Could you check a few things on this model? Use its own coordinates, in mm. Face numbers are marked on the shaded views. A direction names the side the tool comes from. Give positions to 0.01 mm unless a question says otherwise; leave off trailing zeros. Write each loop counter-clockwise with the first axis right and the second up, starting at its lowest first coordinate (ties: lowest second). Pieces come first, ordered by that corner, then holes. Notation, with made-up numbers: M 29.5,-15 L 66.5,-15 A12 cw 66.5,6 Z; hole C -8.5,6.25 d5. An arc over 180 degrees is marked long. Use one line per item in the form item = value.
from build123d import *

# Parameters (mm, degrees)
F0_R      = 14.5
F1_DEPTH  = 2
F2_R      = 11
F3_DEPTH  = 20
F4_R      = 2.9
F5_DEPTH  = 22.001
F6_W      = 3
F6_H      = 3.4
F7_DEPTH  = 2
F8_R      = 0.8
F9_R      = 0.5
F11_W     = 28.85052
F11_H     = 54.144128
F12_DEPTH = 22.001
F14_W     = 3.5
F14_H     = 9


with BuildPart() as f1:
    # F0 (on Top) → F1 (new body)
    with BuildSketch(Plane.XY):
        Circle(F0_R)
    extrude(amount=F1_DEPTH)

    # F2 (on face) → F3 (join)
    with BuildSketch(Plane.XY.offset(2)):
        Circle(F2_R)
    extrude(amount=F3_DEPTH)

    # F4 (on face) → F5 (cut, through all)
    with BuildSketch(Plane(origin=(0, 0, 0), x_dir=(1, 0, 0), z_dir=(0, 0, -1))):
        Circle(F4_R)
    extrude(amount=-F5_DEPTH, mode=Mode.SUBTRACT)

    # F6 (on face) → F7 (join)
    with BuildSketch(Plane.XY.offset(2)):
        with Locations((0, -11)):
            Rectangle(F6_W, F6_H)
    extrude(amount=F7_DEPTH)

    # F8
    f8_edges = [f1.edges().sort_by_distance(p)[0] for p in [
        (-1.5, -12.7, 3),
        (1.5, -12.7, 3),
    ]]
    fillet(f8_edges, radius=F8_R)

    # F9
    f9_edges = [f1.edges().sort_by_distance(p)[0] for p in [
        (-11, 0, 22),
    ]]
    fillet(f9_edges, radius=F9_R)

    # F11 (on Top) → F12 (cut, through all)
    with BuildSketch(Plane.XY):
        with Locations((-14.42526, 2.568883)):
            Rectangle(F11_W, F11_H)
    extrude(amount=F12_DEPTH, mode=Mode.SUBTRACT)

    # F14 (on Front) → F15 (revolve, cut)
    with BuildSketch(Plane.XZ):
        with Locations((9.25, 13.5)):
            Rectangle(F14_W, F14_H)
    revolve(axis=Axis((0, 0, 13.307823), (0, 0, 1)), mode=Mode.SUBTRACT)


solid = f1.part
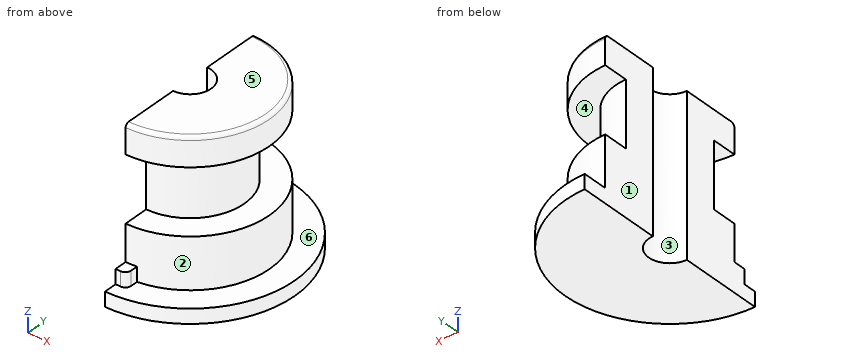
1) I want a section at A-A, the plane y = 0. Please give me the cut outline in (x, z), plus the area to 3 significant figures.
Checked values:
outline = M 2.9,0 L 14.5,0 L 14.5,2 L 11,2 L 11,9 L 7.5,9 L 7.5,18 L 11,18 L 11,21.5 A0.5 ccw 10.5,22 L 2.9,22 Z
area = 154 mm2
2) I want a section at C-C, the plane z = 14. Please give me the cut outline in (x, y).
Checked values:
outline = M 0,-7.5 A7.5 ccw 0,7.5 L 0,2.9 A2.9 cw 0,-2.9 Z
3) Thinking about a two-plate mould opening in Y: for the marked faces 1, 2 and 3, which applies, released by +Y, released by -Y, zero draft, split by the parting line, or undercut?
Checked values:
face_1 = zero draft
face_2 = split by the parting line
face_3 = undercut
4) For the marked faces 4, 5 and 6, which set-ups out of +Z, -Z, +X, -X, +Y, -Y let a thin tool reach every point of the face, with its end or its side?
Checked values:
face_4 = +X
face_5 = +Z, +X, -X, +Y, -Y
face_6 = +Z, +X
5) If I drill on L1, parallel to Z at x = 7.75, y = 2.75; L2, parallel to Z at x = 9, y = -8.75; L3, parallel to Y at x = 4.5, z = 5.75, over which ranges is the centre line in solid material (lowest first)?
Checked values:
L1 = 0 to 9, 18 to 22
L2 = 0 to 2
L3 = -10.04 to 10.04
6) I want a section at B-B, the plane z = 5.5. Please give me the cut outline in (x, y).
Checked values:
outline = M 0,-11 A11 ccw 0,11 L 0,2.9 A2.9 cw 0,-2.9 Z
7) For pin 1 Ø1 at (x, z) = (13, 18.5) entering from -Y; pin 2 Ø6 at (x, y) = (8, 3) entering from -Z; pin 3 Ø6 at (y, z) = (3, 14) entering from +X; pin 4 Ø3 at (y, z) = (-1, 12) entering from -X, each with a flat end and sliding along its axis, tell me the tip position at first contact or that it passes through.
Checked values:
pin_1 = through
pin_2 = 0
pin_3 = 7.5
pin_4 = 1.47
